from build123d import *

# Parameters (mm, degrees)
F0_W     = 609.6
F0_H     = 1219.2
F1_DEPTH = 19.05
F3_DEPTH = 17.145


with BuildPart() as f1:
    # F0 (on Top) → F1 (new body)
    with BuildSketch(Plane.XY):
        Rectangle(F0_W, F0_H)
    extrude(amount=F1_DEPTH)

    # F2 (on face) → F3 (cut)
    with BuildSketch(Plane.XY.offset(19.05)):
        Polygon((304.8, 609.6), (127, 609.6), (127, 139.7), (-304.8, 139.7), (-304.8, 127), (127, 127), (127, -342.9), (-304.8, -342.9), (-304.8, -609.6), (304.8, -609.6), align=None)
    extrude(amount=-F3_DEPTH, mode=Mode.SUBTRACT)


solid = f1.part
For this review, take the finished solid that the model builds, in its own axes (mm). Give positions to 0.01 mm unless a question says otherwise; leave off trailing zeros. Order: outer loops, then holes, each group sorted by start corner. A loop starts at its lowest first (then second) coordinate and runs counter-clockwise, first axis right, second up. Notation, with made-up numbers: M 50.25,76.5 L 105.25,76.5 A22 cw 105.25,106.5 Z; hole C 54,-3 d2. An arc over 180 degrees is marked long. Answer in a Markdown table with one row per item. Add a question column.
(1) For pin 1 (1 mm diameter, centred on x = 238.5, y = 252, fed in from +Z) (3 decimals); pin 2 (8.5 mm diameter, centred on x = 13, z = 7, fed in from -Y); pin 3 (8.5 mm diameter, centred on y = 474.5, z = 13, fed in from +X), all flat-tipped, find the tip position at first contact; note any pin that passes through.
(2) Consider section A-A on z = 12.5. State the section outline as (x, y) points.
(3) Wall thickness on probe 1 along Y at (x, z) = (-242, 2); probe 2 along X at (y, z) = (-291, 6.25); probe 3 along Z at (x, y) = (-260.5, -435) (3 decimals): over which ranges is each line inside the solid? List them lowest first. Write a range as [from, to].
(4) Consider section B-B on x = -207.5. State the section outline as (y, z) points (3 decimals).
(5) Consider section C-C on y = -475.5. State the section outline as (x, z) points (3 decimals).
(6) Consider section D-D on y = -114. State the section outline as (x, z) points (3 decimals).
Evaluation:
| question | item | result |
|---|---|---|
| 1 | pin 1 | stops at z = 1.905 |
| 1 | pin 2 | stops at y = -342.9 |
| 1 | pin 3 | stops at x = 127 |
| 2 | outline | M -304.8,-342.9 L 127,-342.9 L 127,127 L -304.8,127 Z; M -304.8,139.7 L 127,139.7 L 127,609.6 L -304.8,609.6 Z |
| 3 | probe 1 | y = [-342.9, 127], [139.7, 609.6] |
| 3 | probe 2 | x = [-304.8, 127] |
| 3 | probe 3 | z = [0, 1.905] |
| 4 | outline | M -609.6,0 L 609.6,0 L 609.6,19.05 L 139.7,19.05 L 139.7,1.905 L 127,1.905 L 127,19.05 L -342.9,19.05 L -342.9,1.905 L -609.6,1.905 Z |
| 5 | outline | M -304.8,0 L 304.8,0 L 304.8,1.905 L -304.8,1.905 Z |
| 6 | outline | M -304.8,0 L 304.8,0 L 304.8,1.905 L 127,1.905 L 127,19.05 L -304.8,19.05 Z |
